from build123d import *

# Parameters (mm, degrees)
SKETCH1_R           = 4
SKETCH1_R_2         = 1.85
BOSS_EXTRUDE1_DEPTH = 12.5
FILLET1_R           = 10
FILLET2_R           = 3
FILLET3_R           = 10


with BuildPart() as part:
    # Sketch1 → Boss-Extrude1 (new body)
    with BuildSketch(Plane.XY):
        with BuildLine():
            Line((14.142135624, 14.142135624), (28.284271247, 28.284271247))
            ThreePointArc((28.284271247, 28.284271247), (-6.945927107, 39.39231012), (-36.252311481, 16.90473047))
            Line((-36.252311481, 16.90473047), (-45.315389352, 21.130913087))
            ThreePointArc((-45.315389352, 21.130913087), (46.768835106, 17.682648638), (-20, -45.82575695))
            Line((-20, -45.82575695), (-20, 0))
            ThreePointArc((-20, 0), (-7.653668647, 18.47759065), (14.142135624, 14.142135624))
        make_face()
        Circle(SKETCH1_R, mode=Mode.SUBTRACT)
        with Locations((0, 8)):
            Circle(SKETCH1_R_2, mode=Mode.SUBTRACT)
        with Locations((8, 0)):
            Circle(SKETCH1_R_2, mode=Mode.SUBTRACT)
        with Locations((0, -8)):
            Circle(SKETCH1_R_2, mode=Mode.SUBTRACT)
        with Locations((-8, 0)):
            Circle(SKETCH1_R_2, mode=Mode.SUBTRACT)
    extrude(amount=BOSS_EXTRUDE1_DEPTH)

    # Fillet1
    fillet1_edges = [part.edges().sort_by_distance(p)[0] for p in [
        (28.284271247, 28.284271247, 6.25),
        (14.142135624, 14.142135624, 6.25),
    ]]
    fillet(fillet1_edges, radius=FILLET1_R - 0.0001)  # a hair under: the kernel refuses the full size

    # Fillet2
    fillet2_edges = [part.edges().sort_by_distance(p)[0] for p in [
        (-36.252311481, 16.90473047, 6.25),
        (-45.315389352, 21.130913087, 6.25),
    ]]
    fillet(fillet2_edges, radius=FILLET2_R)

    # Fillet3
    fillet3_edges = [part.edges().sort_by_distance(p)[0] for p in [
        (-20, -45.82575695, 6.25),
    ]]
    fillet(fillet3_edges, radius=FILLET3_R)


solid = part.part
Model file for the job. Use its own axes, mm. A direction names the side the tool comes from. Round coordinates to 2 decimals unless told otherwise and drop trailing zeros. Loops run counter-clockwise (first coordinate to the right, second up) from the corner with the lowest first, then second, coordinate; pieces in that order, holes last. Notation, with made-up numbers: (2.5, 17) - (38.5, 17) arc R10 ccw to (38.5, 35) - close; hole circle Ø7 at (41.5, -35). An arc over 180 degrees is marked (long way). Write each question's results on one line, items separated by ' | '.
(1) Saw through at B-B, the plane y = -8. List the corners of the cut face in (x, z), then the cut area to 3 significant figures.
Answer below:
outline: (-20, 0) - (-1.85, 0) - (-1.85, 12.5) - (-20, 12.5) - close; (1.85, 0) - (49.36, 0) - (49.36, 12.5) - (1.85, 12.5) - close | area: 821 mm^2
(2) Pin check, flat tips, straight feed: pin 1 (3 mm diameter, centred on x = 28.5, y = -16, fed in from -Z); pin 2 (6 mm diameter, centred on y = -25.5, z = 5.5, fed in from -X); pin 3 (4 mm diameter, centred on x = -27.5, z = 7, fed in from +Y); pin 4 (5 mm diameter, centred on x = 0, y = 0, fed in from -Z). Stop position of each tip, or through.
Answer below:
pin 1: stops at z = 0 | pin 2: stops at x = -20 | pin 3: stops at y = 43.01 | pin 4: passes through
(3) Saw through at D-D, the plane y = 14. List the corners of the cut face in (x, z).
Answer below:
outline: (-14.28, 0) - (48, 0) - (48, 12.5) - (-14.28, 12.5) - close
(4) Wall check: L1, parallel to Y at x = 0, z = 10.25; L2, parallel to Y at x = 8, z = 3.75; L3, parallel to Y at x = 22, z = 8.25. Give the ranges that are in metal, low to high.
Answer below:
L1: y = -50 to -9.85, -6.15 to -4, 4 to 6.15, 9.85 to 20, 40 to 50 | L2: y = -49.36 to -1.85, 1.85 to 18.33, 39.19 to 49.36 | L3: y = -44.9 to 22.86, 31.28 to 44.9
(5) Mould opens along X. For faces 1 (the cylindrical face through (22.807, 28.63, 6.338)), 2 (the cylindrical face through (-17.849, -44.926, 6.338)), 3 (the cylindrical face through (45.23, 21.31, 6.16)) say: released by +X, released by -X, zero draft, split by the parting line, or undercut.
Answer below:
face 1: undercut | face 2: released by -X | face 3: split by the parting line
(6) Saw through at A-A, the plane x = 0. List the corners of the cut face in (y, z).
Answer below:
outline: (-50, 0) - (-9.85, 0) - (-9.85, 12.5) - (-50, 12.5) - close; (-6.15, 0) - (-4, 0) - (-4, 12.5) - (-6.15, 12.5) - close; (4, 0) - (6.15, 0) - (6.15, 12.5) - (4, 12.5) - close; (9.85, 0) - (20, 0) - (20, 12.5) - (9.85, 12.5) - close; (40, 0) - (50, 0) - (50, 12.5) - (40, 12.5) - close
(7) 3-axis set-ups, long thin cutter, end or side, ignore diameter. For faces 4 (the cylindrical face through (-10.91, 16.76, 6.16)), 5 (the cylindrical face through (-44.08, 21.57, 6.34)), 6 (the flat face through (-20, -20, 6)): which of +Z, -Z, +X, -X, +Y, -Y reach the whole face in a straight line?
Answer below:
face 4: +Z, -Z | face 5: +Z, -Z, -X | face 6: +Z, -Z, -X, -Y
(8) Saw through at C-C, the plane z = 10.25. Count the separate pieces of the cut face and the enclosed holes in it, then the cut area to 3 significant figures.
Answer below:
separate pieces: 1 | enclosed holes: 5 | area: 5,190 mm^2
